Could you check a few things on this model? Use its own coordinates, in mm. A direction names the side the tool comes from. Round coordinates to 2 decimals unless told otherwise and drop trailing zeros. Loops run counter-clockwise (first coordinate to the right, second up) from the corner with the lowest first, then second, coordinate; pieces in that order, holes last. Notation, with made-up numbers: (-27, -13) -> (-19, -13) arc R15 cw to (-19, 2) -> close; hole circle Ø10 at (-26.75, -1.75). An arc over 180 degrees is marked (long way). One line per item, written item: value.
from build123d import *

# Parameters (mm, degrees)
SKETCH1_W           = 10
SKETCH1_H           = 20
SKETCH1_R           = 2.25
BOSS_EXTRUDE1_DEPTH = 4
SKETCH2_W           = 10
SKETCH2_H           = 20
SKETCH2_R           = 4
BOSS_EXTRUDE2_DEPTH = 4


with BuildPart() as part:
    # Sketch1 → Boss-Extrude1 (new body)
    with BuildSketch(Plane(origin=(0, 0, 0), x_dir=(1, 0, 0), z_dir=(0, 1, 0))):
        Rectangle(SKETCH1_W, SKETCH1_H)
        Circle(SKETCH1_R, mode=Mode.SUBTRACT)
    extrude(amount=BOSS_EXTRUDE1_DEPTH)

    # Sketch2 → Boss-Extrude2 (add)
    with BuildSketch(Plane(origin=(0, 4, 0), x_dir=(1, 0, 0), z_dir=(0, 1, 0))):
        Rectangle(SKETCH2_W, SKETCH2_H)
        Circle(SKETCH2_R, mode=Mode.SUBTRACT)
    extrude(amount=BOSS_EXTRUDE2_DEPTH)


solid = part.part
(1) If I drill on L1, parallel to X at y = 1.45, z = 0; L2, parallel to Z at x = 0, y = 5.05; L3, parallel to X at y = 5.9, z = 0, over which ranges is the centre line in solid material (lowest first)?
Recorded:
L1: -5 to -2.25, 2.25 to 5
L2: -10 to -4, 4 to 10
L3: -5 to -4, 4 to 5
(2) Thinking about a two-plate mould opening in X: for faces 3 (the face through (-0.867, 5.972, 3.905)), 4 (the face through (0, 4, -10)), 5 (the face through (-5, 4, 0)), which applies, released by +X, released by -X, zero draft, split by the parting line, or undercut?
Recorded:
face 3: undercut
face 4: zero draft
face 5: released by -X
(3) For faces 1 (the face through (0, 4, 10)), 2 (the face through (2, 4, 2)), which set-ups out of +Z, -Z, +X, -X, +Y, -Y let a thin tool reach every point of the face, with its end or its side?
Recorded:
face 1: +Z, +X, -X, +Y, -Y
face 2: +Y
(4) If we section it at C-C, the plane y = 7.5: Please give me the cut outline in (x, z), then the cut area to 3 significant figures.
Recorded:
outline: (-5, -10) -> (5, -10) -> (5, 10) -> (-5, 10) -> close; hole circle Ø8 at (0, 0)
area: 150 mm²
(5) If we section it at B-B, the plane x = 0: Please give me the cut outline in (y, z).
Recorded:
outline: (0, -10) -> (8, -10) -> (8, -4) -> (4, -4) -> (4, -2.25) -> (0, -2.25) -> close; (0, 2.25) -> (4, 2.25) -> (4, 4) -> (8, 4) -> (8, 10) -> (0, 10) -> close
(6) If we section it at A-A, the plane z = 0: Please give me the cut outline in (x, y), then the cut area to 3 significant figures.
Recorded:
outline: (-5, 0) -> (-2.25, 0) -> (-2.25, 4) -> (-4, 4) -> (-4, 8) -> (-5, 8) -> close; (2.25, 0) -> (5, 0) -> (5, 8) -> (4, 8) -> (4, 4) -> (2.25, 4) -> close
area: 30.0 mm²
(7) I'm going to push a flat-ended pin straight in: pin 1 Ø1 at (x, z) = (4, -3.5) entering from -Y. Where does the tip first touch, or does it pass through?
Recorded:
pin 1: y = 0
(8) If we section it at D-D, the plane x = 3: Please give me the cut outline in (y, z).
Recorded:
outline: (0, -10) -> (8, -10) -> (8, -2.65) -> (4, -2.65) -> (4, 2.65) -> (8, 2.65) -> (8, 10) -> (0, 10) -> close
